Model file for the job. Use its own axes, mm. A direction names the side the tool comes from. Round coordinates to 2 decimals unless told otherwise and drop trailing zeros. Order: outer loops, then holes, each group sorted by start corner. A loop starts at its lowest first (then second) coordinate and runs counter-clockwise, first axis right, second up. Notation, with made-up numbers: M -22.75,62.5 L -16.75,62.5 A26 cw -16.75,97.5 Z; hole C 71,-12 d5. An arc over 180 degrees is marked long. Return JSON: item names as keys, results as strings. Group by question number.
Item 1: Pull direction Z, two halves, no side cores. Call faces 4 (the face through (-4.036, -30.736, 1.014)), 5 (the face through (-8, -19, 5)), 6 (the face through (-7, 27.4, 8)), 7 (the face through (25.865, 10.724, 4.281)): pulls with the +Z half, pulls with the -Z half, needs draft (parallel to the pull), parting line crosses it, or undercut.
Item 2: Slice it at D-D on z = 37.5. Write the cut outline in (x, y).
Item 3: Probe line 1 along X through (y, z) = (17, 27); line 2 along Z through (x, y) = (14.5, 25); line 3 along Y through (x, z) = (-8, 3). List the from-to ranges inside material, lowest first.
Item 4: Pin check, flat tips, straight feed: pin 1 Ø11 at (y, z) = (2.5, 14) entering from -X; pin 2 Ø1.5 at (x, z) = (13, 33.5) entering from -Y; pin 3 Ø8 at (x, z) = (2.5, 18) entering from -Y. Stop position of each tip, or through.
Item 5: Slice it at B-B on y = 0. Give the number of separate pieces and of enclosed holes in the cut face, then the cut area to 3 significant figures.
Item 6: Slice it at A-A on z = 9.5. Write the cut outline in (x, y), then the cut area to 3 significant figures.
Item 7: Which spindle directions (+Z, -Z, +X, -X, +Y, -Y) get a long thin tool onto all of the face, cutting with end or side? Do faces 1 (the face through (-16.61, -7.28, 19.79)), 2 (the face through (-20.2, 2.4, 2.5)), 3 (the face through (25.865, 10.724, 20.422)). Say none if no direction does.
from build123d import *

# Parameters (mm, degrees)
F0_W     = 23
F0_H     = 5
F2_R     = 4
F3_DEPTH = 5
F6_DEPTH = 25
F7_DEPTH = 35
F5_DEPTH = 35
F8_COUNT = 6


with BuildPart() as f1:
    # F0 (on Front) → F1 (revolve)
    with BuildSketch(Plane.XZ):
        with Locations((11.5, 2.5)):
            Rectangle(F0_W, F0_H)
        Polygon((23, 5), (23, 0), (31, 0), (31, 2), (28, 2), (28, 6.5), (31, 6.5), (31, 8), (28, 8), (28, 32.5), (31, 32.5), (31, 34), (28, 34), (28, 38.5), (31, 38.5), (31, 40.5), (23, 40.5), (23, 20.25), align=None)
    revolve(axis=Axis((0, 0, 2.5), (0, 0, -1)))

    # F2 (on face) → F3 (cut, through all)
    with BuildSketch(Plane(origin=(0, 0, 0), x_dir=(1, 0, 0), z_dir=(0, 0, -1))):
        with Locations((-17, 0)):
            Circle(F2_R)
        with Locations((-8.5, -14.7224318643)):
            Circle(F2_R)
        with Locations((8.5, -14.7224318643)):
            Circle(F2_R)
        with Locations((17, 0)):
            Circle(F2_R)
        with Locations((8.5, 14.7224318643)):
            Circle(F2_R)
        with Locations((-8.5, 14.7224318643)):
            Circle(F2_R)
    extrude(amount=-F3_DEPTH, mode=Mode.SUBTRACT)

    # F4 (on Top) → F6 (join)
    with BuildSketch(Plane.XY):
        Polygon((8.5, 4.9074772881), (0, 9.8149545762), (-8.5, 4.9074772881), (-8.5, -4.9074772881), (0, -9.8149545762), (8.5, -4.9074772881), align=None)
    extrude(amount=F6_DEPTH)

    # F4 (on Top) → F7 (join)
    with BuildSketch(Plane.XY):
        Polygon((2, 9.8149545762), (0, 9.8149545762), (-2, 9.8149545762), (-2, 13.2790561914), (-12.5, 7.2168783649), (-12.5, -7.2168783649), (0, -14.4337567297), (12.5, -7.2168783649), (12.5, 7.2168783649), (2, 13.2790561914), align=None)
        Polygon((-8.5, 4.9074772881), (0, 9.8149545762), (8.5, 4.9074772881), (8.5, -4.9074772881), (0, -9.8149545762), (-8.5, -4.9074772881), align=None, mode=Mode.SUBTRACT)
        Polygon((-2, 9.8149545762), (0, 9.8149545762), (2, 9.8149545762), (2, 13.2790561914), (0, 14.4337567297), (-2, 13.2790561914), align=None)
    extrude(amount=F7_DEPTH)

    # F4 (on Top) → F5 (join)
    with BuildSketch(Plane.XY):
        Polygon((-2, 23), (-2, 13.2790561914), (0, 14.4337567297), (2, 13.2790561914), (2, 23), align=None)
    extrude(amount=F5_DEPTH)

    # F8: F1 ×6 about axis
    f8_axis = Axis((0, 0, 40.5), (0, 0, -1))


with BuildPart() as f1_1:
    add(f1.part)
    for i in range(1, F8_COUNT):
        add(f1.part.rotate(f8_axis, i * 360 / F8_COUNT))


solid = f1_1.part
Output values:
{
 "1": {"face 4": "needs draft", "face 5": "pulls with the +Z half", "face 6": "undercut", "face 7": "undercut"},
 "2": {"outline": "C 0,0 d56; hole C 0,0 d46"},
 "3": {"line 1": "-22.25 to -15.49, -2 to 2, 15.49 to 22.25", "line 2": "0 to 2, 6.5 to 8, 32.5 to 34, 38.5 to 40.5", "line 3": "-26.83 to -18.69, -10.75 to 10.75, 18.69 to 26.83"},
 "4": {"pin 1": "x = -28", "pin 2": "y = -28.48", "pin 3": "y = -28"},
 "5": {"separate pieces": "3", "enclosed holes": "0", "area": "1,180 mm²"},
 "6": {"outline": "C 0,0 d56; hole M -20.84,-9.72 L -12.5,-4.91 L -12.5,4.91 L -20.84,9.72 A23 ccw Z; hole M -18.84,-13.19 A23 ccw -2,-22.91 L -2,-13.28 L -10.5,-8.37 Z; hole M -18.84,13.19 L -10.5,8.37 L -2,13.28 L -2,22.91 A23 ccw Z; hole M 2,-22.91 A23 ccw 18.84,-13.19 L 10.5,-8.37 L 2,-13.28 Z; hole M 2,13.28 L 10.5,8.37 L 18.84,13.19 A23 ccw 2,22.91 Z; hole M 12.5,-4.91 L 20.84,-9.72 A23 ccw 20.84,9.72 L 12.5,4.91 Z", "area": "1,560 mm²"},
 "7": {"face 1": "+Z", "face 2": "+Z, -Z", "face 3": "none"}
}
